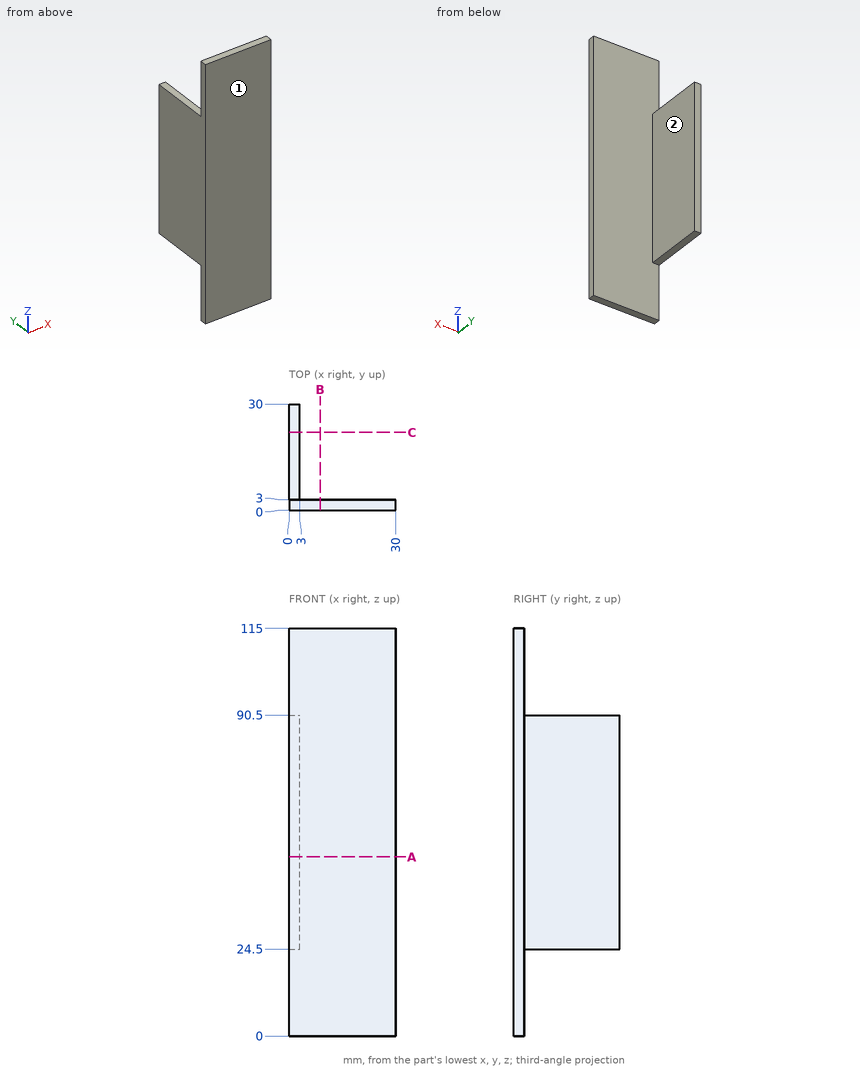
Answer from the drawing. Dimensions are ordinates in mm from the lowest x, y and z of the part. A direction names the side the tool comes from. Round coordinates to 2 decimals unless told otherwise and drop trailing zeros. Loops run counter-clockwise (first coordinate to the right, second up) from the corner with the lowest first, then second, coordinate; pieces in that order, holes last. Notation, with made-up numbers: (-39, 46) - (-30, 46) arc R22 ccw to (-30, 71) - close; hole circle Ø7 at (75.5, -14.5). An arc over 180 degrees is marked (long way). Return JSON: item names as keys, results as strings. Group by question number.
1. Each of these flat-tipped pins is pushed along its axis until it touches: P1, Ø1, axis at x = 15.5, y = 4, coming from the -Z side; P2, Ø2.5, axis at x = 1.5, y = 21.5, coming from the +Z side; P3, Ø3.5, axis at x = 1, y = 15, coming from the -Z side; P4, Ø9, axis at x = 12, z = 61, coming from the +Y side. Where does it stop, or does it pass through?
2. The part is cut by section B-B on x = 8.75. Determine the outline of the cut face in (y, z), then the cut area to 3 significant figures.
3. Which of the six approach directions +Z, -Z, +X, -X, +Y, -Y give full straight-line access (tool end or side, diameter ignored) to the marked faces 1 and 2?
4. The part is cut by section A-A on z = 50.5. Determine the outline of the cut face in (x, y).
5. Consider probe 1 along Y at (x, z) = (10, 61.5). Determine where the line is inside the solid, lowest interval first.
6. The part is cut by section C-C on y = 22. Determine the outline of the cut face in (x, z), then the cut area to 3 significant figures.
Resolved:
{
 "1": {"P1": "passes through", "P2": "stops at z = 90.5", "P3": "stops at z = 24.5", "P4": "stops at y = 3"},
 "2": {"outline": "(0, 0) - (3, 0) - (3, 115) - (0, 115) - close", "area": "345 mm²"},
 "3": {"face 1": "+Z, -Z, +X, -X, -Y", "face 2": "+Z, -Z, +X, +Y"},
 "4": {"outline": "(0, 0) - (30, 0) - (30, 3) - (3, 3) - (3, 30) - (0, 30) - close"},
 "5": {"probe 1": "y = 0 to 3"},
 "6": {"outline": "(0, 24.5) - (3, 24.5) - (3, 90.5) - (0, 90.5) - close", "area": "198 mm²"}
}
